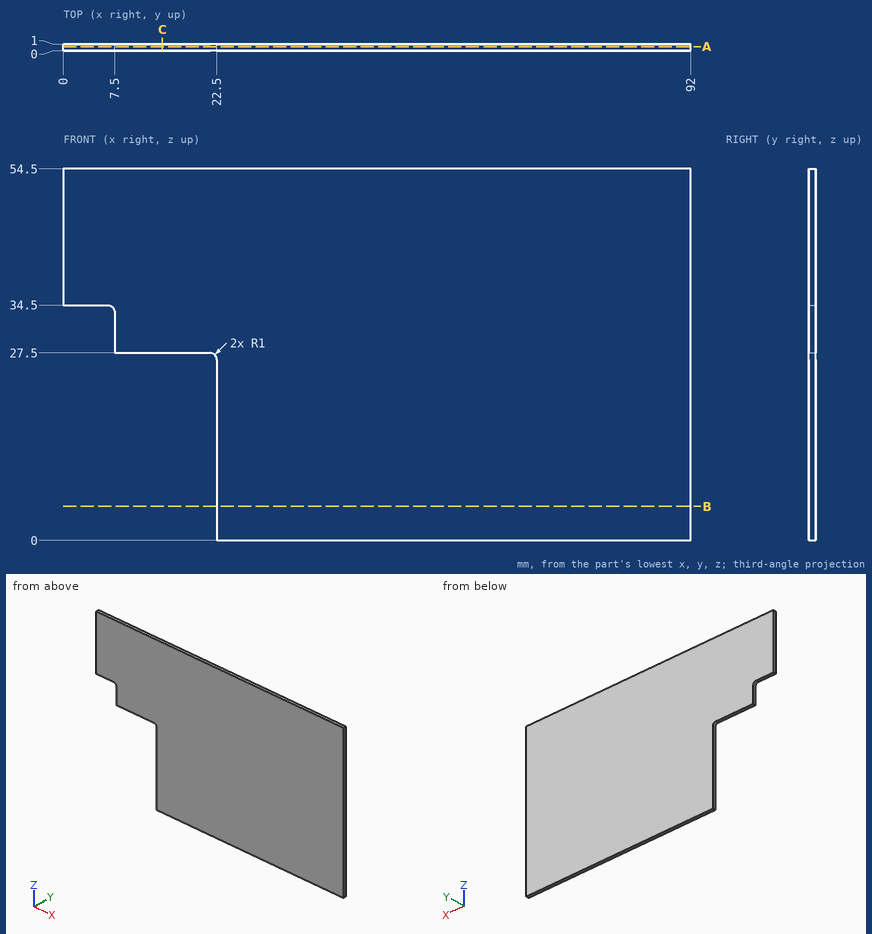
The drawing under review shows one solid part. Ordinate dimensions are in mm from its lowest x, y, z. Give positions to 0.01 mm unless a question says otherwise; leave off trailing zeros. Order: outer loops, then holes, each group sorted by start corner. A loop starts at its lowest first (then second) coordinate and runs counter-clockwise, first axis right, second up. Notation, with made-up numbers: (47.5, 9.5) - (59.5, 9.5) arc R19 ccw to (59.5, 28.5) - close; hole circle Ø8 at (47, 75.25). An arc over 180 degrees is marked (long way). Answer as a JSON object with one key per item and string values. Group by question number.
Item 1: Wall thickness on line 1 along Z through (x, y) = (14.5, 0.9); line 2 along X through (y, z) = (0.3, 33); line 3 along X through (y, z) = (0.65, 26.5): over which ranges is each line inside the solid? List them lowest first.
Item 2: Take a section at C-C on x = 14.5. Give the boundary of the cut face in (y, z).
Item 3: Take a section at A-A on y = 0.6. Give the boundary of the cut face in (x, z), and give its area (3 significant figures).
Item 4: Take a section at B-B on z = 5. Give the boundary of the cut face in (x, y), and give its area (3 significant figures).
Reported:
{
 "1": {"line 1": "27.5 to 54.5", "line 2": "7.5 to 92", "line 3": "22.5 to 92"},
 "2": {"outline": "(0, 27.5) - (1, 27.5) - (1, 54.5) - (0, 54.5) - close"},
 "3": {"outline": "(0, 34.5) - (6.5, 34.5) arc R1 cw to (7.5, 33.5) - (7.5, 27.5) - (21.5, 27.5) arc R1 cw to (22.5, 26.5) - (22.5, 0) - (92, 0) - (92, 54.5) - (0, 54.5) - close", "area": "4,340 mm^2"},
 "4": {"outline": "(22.5, 0) - (92, 0) - (92, 1) - (22.5, 1) - close", "area": "69.5 mm^2"}
}
